Here's the drawing with two shaded views (mm, measured from the low corner). I have some questions. A direction names the side the tool comes from. Coordinates: 2 decimals unless noted, no trailing zeros. Write each loop counter-clockwise with the first axis right and the second up, starting at its lowest first coordinate (ties: lowest second). Pieces come first, ordered by that corner, then holes.
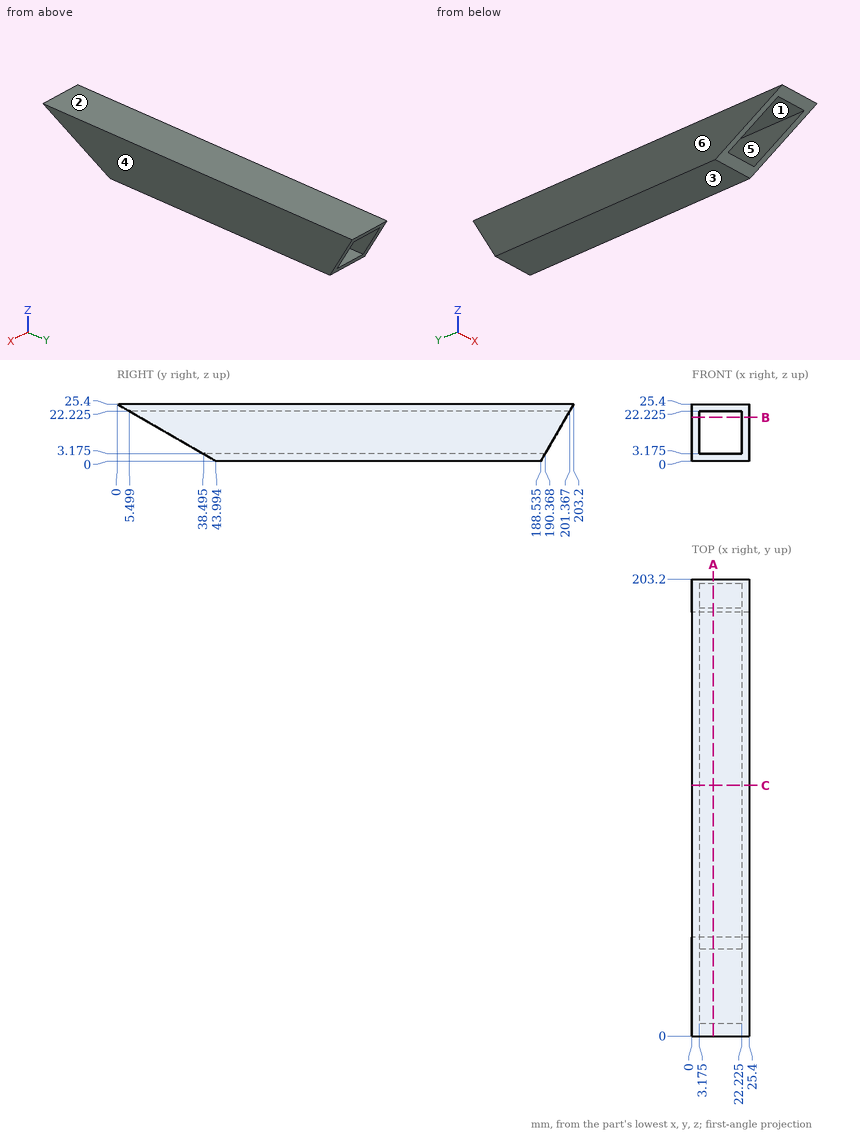
1. I want a section at C-C on y = 111.5. Please give me the cut outline in (x, z) (1 decimal), plus the area to 3 significant figures.
Verdict:
outline: (0, 0) - (25.4, 0) - (25.4, 25.4) - (0, 25.4) - close; hole (3.2, 3.2) - (22.2, 3.2) - (22.2, 22.2) - (3.2, 22.2) - close
area: 282 mm2
2. If we mould it in two halves opening along Z, with no side actions, what happens to the marked faces 1, 2, 3 and 4? For each: pulls with the +Z half, pulls with the -Z half, needs draft (parallel to the pull), parting line crosses it, or undercut.
Verdict:
face 1: undercut
face 2: pulls with the +Z half
face 3: pulls with the -Z half
face 4: needs draft
3. I want a section at B-B on z = 19.5. Please give me the cut outline in (x, y) (1 decimal), plus the area to 3 significant figures.
Verdict:
outline: (0, 10.2) - (3.2, 10.2) - (3.2, 199.8) - (0, 199.8) - close; (22.2, 10.2) - (25.4, 10.2) - (25.4, 199.8) - (22.2, 199.8) - close
area: 1,200 mm2
4. I want a section at A-A on x = 9.5. Please give me the cut outline in (y, z) (1 decimal), plus the area to 3 significant figures.
Verdict:
outline: (0, 25.4) - (5.5, 22.2) - (201.4, 22.2) - (203.2, 25.4) - close; (38.5, 3.2) - (44, 0) - (188.5, 0) - (190.4, 3.2) - close
area: 1,100 mm2
5. On a 3-axis mill with a long thin cutter (end or side, diameter ignored), from which of +Z, -Z, +X, -X, +Y, -Y can I reach the whole of each face in a straight line? I mean the marked faces 5 and 6. Say none if no direction works.
Verdict:
face 5: +Y, -Y
face 6: +Z, -Z, -X, +Y, -Y
6. Please list where these lines run through material, in increasing order: line 1 along Z through (x, y) = (21.25, 78) (1 decimal); line 2 along Z through (x, y) = (12, 30) (1 decimal).
Verdict:
line 1: z = 0 to 3.2, 22.2 to 25.4
line 2: z = 22.2 to 25.4
7. For pin 1 (6 mm diameter, centred on x = 15.5, z = 8, fed in from -Y); pin 2 (8 mm diameter, centred on x = 8.5, y = 30, fed in from -Z) (3 decimals); pin 3 (1.5 mm diameter, centred on x = 3.5, z = 22, fed in from +Y), each with a flat end and sliding along its axis, tell me the tip position at first contact or that it passes through.
Verdict:
pin 1: passes through
pin 2: stops at z = 22.225
pin 3: stops at y = 201.67
